```python
from build123d import *

# Parameters (mm, degrees)
F1_DEPTH = 2
F0_R     = 11.5
F2_DEPTH = 2


# Not quite as in the source:
# - a feature names something its author has since deleted; it is built from what else it names


with BuildPart() as f1:
    # F0 (on Front) → F1 (new body)
    with BuildSketch(Plane.XZ):
        with BuildLine():
            Line((-1.9, -2.19089023), (-1.9, 2.19089023))
            ThreePointArc((-1.9, 2.19089023), (-2.9, 0), (-1.9, -2.19089023))
        make_face()
    extrude(amount=F1_DEPTH)



with BuildPart() as f1b:
    # F0 (on Front) → F1, piece 2 (new body)
    with BuildSketch(Plane.XZ):
        with BuildLine():
            ThreePointArc((1.9, -2.19089023), (2.6381811917, -1.2041594579), (2.9, 0))
            ThreePointArc((2.9, 0), (2.6381811917, 1.2041594579), (1.9, 2.19089023))
            Line((1.9, 2.19089023), (1.9, -2.19089023))
        make_face()
    extrude(amount=F1_DEPTH)


with BuildPart() as f1_1:
    add(f1.part)

    add(f1b.part)  # F2 merges F1b
    # F0 (on Front) → F2 (join)
    with BuildSketch(Plane.XZ):
        Circle(F0_R)
        with BuildLine():
            ThreePointArc((1.9, 2.19089023), (2.6381811917, 1.2041594579), (2.9, 0))
            ThreePointArc((2.9, 0), (2.6381811917, -1.2041594579), (1.9, -2.19089023))
            ThreePointArc((1.9, -2.19089023), (0, -2.9), (-1.9, -2.19089023))
            ThreePointArc((-1.9, -2.19089023), (-2.9, 0), (-1.9, 2.19089023))
            ThreePointArc((-1.9, 2.19089023), (0, 2.9), (1.9, 2.19089023))
        make_face(mode=Mode.SUBTRACT)
    extrude(amount=F2_DEPTH)


solid = f1_1.part
```
Source: CAD feature listing. Evaluate the final solid. Frame: model axes, mm. A direction names the side the tool comes from. Coordinates: 2 decimals unless noted, no trailing zeros. Loops run counter-clockwise (first coordinate to the right, second up) from the corner with the lowest first, then second, coordinate; pieces in that order, holes last. Notation, with made-up numbers: M -9.5,-38.5 L 38.5,-38.5 A21 ccw 38.5,-15.5 Z; hole C 12.5,59.5 d10. An arc over 180 degrees is marked long. Use a Markdown table: item, result. Add a question column.
Q1. Material intervals for L1, parallel to X at y = -1.15, z = -2; L2, parallel to X at y = -0.3, z = 0.5; L3, parallel to Z at x = 9.75, y = -0.7, sorted ascending.
Q2. Access query for faces 4 (the cylindrical face through (0, -1, 2.9)), 5 (the flat face through (2.4, 0, 0.2)). Directions: +Z, -Z, +X, -X, +Y, -Y. A direction counts if a zero-diameter tool reaches every point of the face in a straight line with its end or side. Return the directions, or none.
Q3. Section query D-D, the plane x = -3.75. Return loops of the section in (y, z), and give its area (3 significant figures).
Q4. Section query C-C, the plane y = -1.45. Return loops of the section in (x, z), and give its area (3 significant figures).
Q5. Draft query along X for faces 1 (the flat face through (2.4, -2, 0.2)), 2 (the cylindrical face through (0, -1, -2.9)), 3 (the cylindrical face through (-1.5, -1, 11.4)). Return one class per face: pulls with the +X half, pulls with the -X half, needs draft (parallel to the pull), parting line crosses it, or undercut.
Q6. Section query A-A, the plane x = 0. Return loops of the section in (y, z).
Q7. Section query B-B, the plane z = 0. Return loops of the section in (x, y).
Result:
| question | item | result |
|---|---|---|
| 1 | L1 | x = -11.32 to -1.9, 1.9 to 11.32 |
| 1 | L2 | x = -11.49 to -1.9, 1.9 to 11.49 |
| 1 | L3 | z = -6.1 to 6.1 |
| 2 | face 4 | +Y, -Y |
| 2 | face 5 | +Z, -Z, +X, -X, +Y |
| 3 | outline | M -2,-10.87 L 0,-10.87 L 0,10.87 L -2,10.87 Z |
| 3 | area | 43.5 mm2 |
| 4 | outline | C 0,0 d23; hole M -1.9,-2.19 A2.9 ccw 1.9,-2.19 L 1.9,2.19 A2.9 ccw -1.9,2.19 Z |
| 4 | area | 395 mm2 |
| 5 | face 1 | needs draft |
| 5 | face 2 | undercut |
| 5 | face 3 | parting line crosses it |
| 6 | outline | M -2,-11.5 L 0,-11.5 L 0,-2.9 L -2,-2.9 Z; M -2,2.9 L 0,2.9 L 0,11.5 L -2,11.5 Z |
| 7 | outline | M -11.5,-2 L -1.9,-2 L -1.9,0 L -11.5,0 Z; M 1.9,-2 L 11.5,-2 L 11.5,0 L 1.9,0 Z |
